Here's how the part is built. I have some questions about the finished solid (model axes, mm). Face numbers are marked on the shaded views. A direction names the side the tool comes from. Coordinates: 2 decimals unless noted, no trailing zeros. Write each loop counter-clockwise with the first axis right and the second up, starting at its lowest first coordinate (ties: lowest second). Pieces come first, ordered by that corner, then holes.
Item 1: We'd pull the mould along X, two halves only. Please class the marked faces 5, 6, 7 and 8: +X half, -X half, draft (parallel to the pull), parting line (faces both ways), or undercut.
Item 2: If we section it at D-D (x = -462): Please give me the cut outline in (y, z), then the cut area to 3 significant figures.
Item 3: If I drill on line 1 (X direction, y = -55, z = 2.75); line 2 (Y direction, x = -435, z = 14); line 3 (X direction, y = -170, z = 18.75), over which ranges is the centre line in solid material (lowest first)?
Item 4: For the marked faces 1, 2, 3 and 4, which set-ups out of +Z, -Z, +X, -X, +Y, -Y let a thin tool reach every point of the face, with its end or its side?
Item 5: I'm going to push flat-ended pins straight in: pin 1 Ø12 at (x, z) = (-436.5, 18.5) entering from -Y; pin 2 Ø1 at (x, y) = (-461, -136) entering from -Z; pin 3 Ø7.5 at (y, z) = (-83, 11) entering from +X; pin 4 Ø10 at (y, z) = (-137, 9) entering from +X. Where does each tip first touch, or does it pass through?
Item 6: If we section it at A-A (y = -98): Please give me the cut outline in (x, z), then the cut area to 3 significant figures.
Item 7: If we section it at B-B (x = -410): Please give me the cut outline in (y, z), then the cut area to 3 significant figures.
Item 8: If we section it at C-C (y = -65): Please give me the cut outline in (x, z), then the cut area to 3 significant figures.
from build123d import *

# Parameters (mm, degrees)
F1_DEPTH = 25.4


with BuildPart() as f1:
    # F0 (on Top) → F1 (new body)
    with BuildSketch(Plane.XY):
        with BuildLine():
            add(Edge.make_bspline(
                [(-480.5364153451, -139.2066991603), (-475.5801438199, -132.1421628818), (-465.4086910628, -120.7131486929)],
                knots=[0, 0, 0, 1, 1, 1], degree=2))
            Line((-480.5364153451, -139.2066991603), (-481.4610928685, -139.2066991603))
            add(Edge.make_bspline(
                [(-480.5364153451, -119.566548564), (-480.5364153451, -125.8913428238), (-481.4610928685, -139.2066991603)],
                knots=[0, 0, 0, 1, 1, 1], degree=2))
            Line((-480.5364153451, -119.566548564), (-480.5364153451, -24.1768152531))
            Line((-480.5364153451, -24.1768152531), (-499.5107981247, -24.1768152531))
            Line((-499.5107981247, -24.1768152531), (-499.5107981247, -204.0450870991))
            Line((-499.5107981247, -204.0450870991), (-480.5364153451, -204.0450870991))
            Line((-480.5364153451, -204.0450870991), (-480.5364153451, -156.6646108016))
            Line((-480.5364153451, -156.6646108016), (-466.1114459806, -144.1629706856))
            Line((-466.1114459806, -144.1629706856), (-421.3570538494, -204.0450870991))
            Line((-421.3570538494, -204.0450870991), (-398.1291544624, -204.0450870991))
            Line((-398.1291544624, -204.0450870991), (-453.0549993506, -131.3284466612))
            Line((-453.0549993506, -131.3284466612), (-401.716903253, -77.3642663973))
            Line((-401.716903253, -77.3642663973), (-424.5009574289, -77.3642663973))
            Line((-424.5009574289, -77.3642663973), (-465.4086910628, -120.7131486929))
        make_face()
    extrude(amount=F1_DEPTH)


solid = f1.part
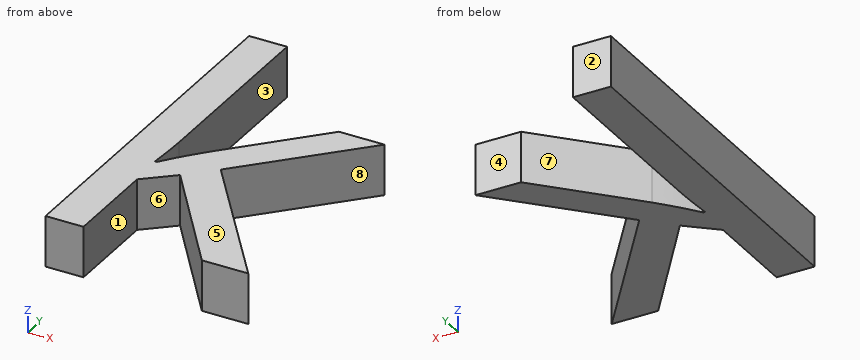
Answer list:
1. face 5: draft
1. face 6: undercut
1. face 7: undercut
1. face 8: +X half
2. outline: (-149.66, 0) - (-117.1, 0) - (-117.1, 25.4) - (-149.66, 25.4) - close
2. area: 827 mm2
3. line 1: x = -499.51 to -480.54
3. line 2: y = -185.79 to -155.23, -112.35 to -88.49
3. line 3: x = -499.51 to -480.54, -446.8 to -423.84
4. face 1: +Z, -Z, -Y
4. face 2: +Z, -Z, +X, -X, +Y
4. face 3: +Z, -Z, +Y
4. face 4: +Z, -Z, +X, +Y
5. pin 1: stops at y = -191.81
5. pin 2: stops at z = 0
5. pin 3: stops at x = -403.51
5. pin 4: stops at x = -444.99
6. outline: (-499.51, 0) - (-480.54, 0) - (-480.54, 25.4) - (-499.51, 25.4) - close; (-443.97, 0) - (-421.35, 0) - (-421.35, 25.4) - (-443.97, 25.4) - close
6. area: 1,060 mm2
7. outline: (-204.05, 0) - (-188.33, 0) - (-188.33, 25.4) - (-204.05, 25.4) - close; (-86.07, 0) - (-77.36, 0) - (-77.36, 25.4) - (-86.07, 25.4) - close
7. area: 620 mm2
8. outline: (-499.51, 0) - (-480.54, 0) - (-480.54, 25.4) - (-499.51, 25.4) - close
8. area: 482 mm2
